```python
from build123d import *

# Parameters (mm, degrees)
F0_R     = 3.3666282328
F0_R_2   = 4.2780726565
F1_DEPTH = 25.4


with BuildPart() as f1:
    # F0 (on Top) → F1 (new body)
    with BuildSketch(Plane.XY):
        with BuildLine():
            ThreePointArc((-22.1343814945, 32.3195395849), (-10.7773284043, 37.9899650978), (-6.1959977362, 49.8283682714))
            ThreePointArc((-6.1959977362, 49.8283682714), (-8.017979687, 57.6234855899), (-13.1064001471, 63.8034086848))
            ThreePointArc((-13.1064001471, 63.8034086848), (-15.7610771081, 65.4788003499), (-18.6713267733, 66.6555305166))
            ThreePointArc((-18.6713267733, 66.6555305166), (-25.3338728535, 67.3459786854), (-31.771318173, 65.4951581371))
            ThreePointArc((-31.771318173, 65.4951581371), (-34.6785879171, 63.6321004456), (-37.1657780069, 61.236878789))
            ThreePointArc((-37.1657780069, 61.236878789), (-39.9749449815, 42.9676641594), (-24.8959708176, 32.2774742434))
            ThreePointArc((-24.8959708176, 32.2774742434), (-23.515806874, 32.3399135434), (-22.1343814945, 32.3195395849))
        make_face()
        with Locations((-33.5280001163, 56.845203042)):
            Circle(F0_R, mode=Mode.SUBTRACT)
        with Locations((-18.897600472, 56.845203042)):
            Circle(F0_R_2, mode=Mode.SUBTRACT)
        with BuildLine():
            ThreePointArc((-18.6713267733, 66.6555305166), (-15.7610771081, 65.4788003499), (-13.1064001471, 63.8034086848))
            Line((-13.1064001471, 63.8034086848), (-13.1064001471, 73.6092031002))
            Line((-13.1064001471, 73.6092031002), (-18.6713267733, 66.6555305166))
        make_face()
        with BuildLine():
            ThreePointArc((-3.572438767, 21.4317220567), (-11.5045727225, 29.1751773236), (-22.1343814945, 32.3195395849))
            ThreePointArc((-22.1343814945, 32.3195395849), (-23.5143490847, 32.2442096875), (-24.8959708176, 32.2774742434))
            ThreePointArc((-24.8959708176, 32.2774742434), (-35.1264416512, 28.9952801275), (-42.7571638322, 21.4317220567))
            ThreePointArc((-42.7571638322, 21.4317220567), (-29.4734249224, -12.8695185824), (-0.1186150736, 9.2964004725))
            ThreePointArc((-0.1186150736, 9.2964004725), (-0.9988822447, 15.6050240953), (-3.572438767, 21.4317220567))
        make_face()
        with BuildLine():
            ThreePointArc((-24.8959708176, 32.2774742434), (-23.5143490847, 32.2442096875), (-22.1343814945, 32.3195395849))
            ThreePointArc((-22.1343814945, 32.3195395849), (-23.515806874, 32.3399135434), (-24.8959708176, 32.2774742434))
        make_face()
        with BuildLine():
            ThreePointArc((-37.1657780069, 61.236878789), (-34.6785879171, 63.6321004456), (-31.771318173, 65.4951581371))
            Line((-31.771318173, 65.4951581371), (-37.1657780069, 70.8660041886))
            Line((-37.1657780069, 70.8660041886), (-37.1657780069, 61.236878789))
        make_face()
        with Locations((-33.5280001163, 56.845203042)):
            Circle(F0_R)
        with Locations((-18.897600472, 56.845203042)):
            Circle(F0_R_2)
    extrude(amount=F1_DEPTH)


solid = f1.part
```
For this review, take the finished solid that the model builds, in its own axes (mm). A direction names the side the tool comes from. Round coordinates to 2 decimals unless told otherwise and drop trailing zeros. Write each loop counter-clockwise with the first axis right and the second up, starting at its lowest first coordinate (ties: lowest second). Pieces come first, ordered by that corner, then holes. Notation, with made-up numbers: M 15,26 L 23,26 A20 cw 23,61 Z; hole C 87,37 d1. An arc over 180 degrees is marked long. One line per item, written item: value. Start each with the question number.
(1) We need section C-C (x = -28). Give the boundary of the cut face in (y, z).
(2) The part is to be moulded in two halves that separate along X. For faces 1 (the flat face through (-23, 21, 25.4)), 2 (the flat face through (-37.166, 66, 13)), 3 (the cylindrical face through (-25.24, 67.354, 12.522)), say which applies: released by +X, released by -X, zero draft, split by the parting line, or undercut.
(3) We need section B-B (z = 5). Give the boundary of the cut face in (x, y).
(4) Insertion check: pin 1 (12 mm diameter, centred on x = -5, y = 27.5, fed in from -Z); pin 2 (2 mm diameter, centred on x = -6, z = 15, fed in from -Y); pin 3 (8 mm diameter, centred on y = 18.5, z = 22.5, fed in from +X); pin 4 (2 mm diameter, centred on y = 45, z = 12.5, fed in from +X). Each pin has a flat end and moves straight along its axis. Give the tip position at first contact, or say it passes through.
(5) We need section A-A (x = -8.5). Give the boundary of the cut face in (y, z), and give its area (3 significant figures).
(6) Machinability: for faces 4 (the flat face through (-23, 21, 0)), 5 (the flat face through (-15.85, 70.18, 12.52)), 6 (the flat face through (-13.106, 69, 13)), which of the approach directions +Z, -Z, +X, -X, +Y, -Y give a long, thin tool a straight path to every point of the face, cutting with its end or side? Answer none if there is none.
(7) Wall thickness on line 1 (Y direction, x = -38, z = 13.5); line 2 (Y direction, x = -34.5, z = 13.75); line 3 (Y direction, x = -23.5, z = 5.75): over which ranges is each line inside the solid? List them lowest first.
(8) We need section D-D (y = 45.5). Give the boundary of the cut face in (x, z), and give its area (3 significant figures).
Result:
1. outline: M -13.24,0 L 31.83,0 L 31.83,25.4 L -13.24,25.4 Z; M 32.76,0 L 66.9,0 L 66.9,25.4 L 32.76,25.4 Z
2. face 1: zero draft
2. face 2: released by -X
2. face 3: undercut
3. outline: M -37.17,61.24 A17.59 ccw -24.9,32.28 A23.05 ccw long -22.13,32.32 A17.59 ccw -13.11,63.8 L -13.11,73.61 L -18.67,66.66 A17.59 ccw -31.77,65.5 L -37.17,70.87 Z
4. pin 1: z = 0
4. pin 2: y = -7.13
4. pin 3: x = -0.71
4. pin 4: x = -6.62
5. outline: M -8.48,0 L 27.07,0 L 27.07,25.4 L -8.48,25.4 Z; M 41.13,0 L 58.53,0 L 58.53,25.4 L 41.13,25.4 Z
5. area: 1,350 mm²
6. face 4: -Z, +X, -X, +Y, -Y
6. face 5: +Z, -Z, +Y
6. face 6: +Z, -Z, +X, +Y
7. line 1: -8.34 to 26.93, 39.48 to 60.18
7. line 2: -10.77 to 29.36, 35.89 to 68.21
7. line 3: -13.75 to 67.41
8. outline: M -40.83,0 L -6.74,0 L -6.74,25.4 L -40.83,25.4 Z
8. area: 866 mm²
